```python
from build123d import *

# Parameters (mm, degrees)
EXTRUDE_1_DEPTH     = 10
CUT_EXTRUDE_1_REACH = 42.24
SKETCH_2_W          = 5
SKETCH_2_H          = 10


with BuildPart() as part:
    # 草圖1 → 伸長1 (new body)
    with BuildSketch(Plane.XY):
        with BuildLine():
            Line((-466, 20.12), (466, 20.12))
            ThreePointArc((466, 20.12), (486.12, 0), (466, -20.12))
            Line((466, -20.12), (-466, -20.12))
            ThreePointArc((-466, -20.12), (-486.12, 0), (-466, 20.12))
        make_face()
        with BuildLine():
            Line((-466, 18.62), (466, 18.62))
            ThreePointArc((466, 18.62), (484.62, 0), (466, -18.62))
            Line((466, -18.62), (-466, -18.62))
            ThreePointArc((-466, -18.62), (-484.62, 0), (-466, 18.62))
        make_face(mode=Mode.SUBTRACT)
    extrude(amount=EXTRUDE_1_DEPTH)

    # 草圖2 → 除料-伸長1 (cut, up to next)
    with BuildSketch(Plane(origin=(0, 20.12, 0), x_dir=(1, 0, 0), z_dir=(0, 1, 0)), mode=Mode.PRIVATE) as cut_extrude_1_sk1:
        with Locations((27.677656209, -5)):
            Rectangle(SKETCH_2_W, SKETCH_2_H)
    cut_extrude_1_tool1 = extrude(cut_extrude_1_sk1.sketch, amount=-CUT_EXTRUDE_1_REACH, mode=Mode.PRIVATE) & part.part
    add(cut_extrude_1_tool1.solids().sort_by_distance((27.677656, 20.12, 5))[0], mode=Mode.SUBTRACT)


solid = part.part
```
Verification items for the finished model (mm, model axes). A direction names the side the tool comes from. Coordinates: 2 decimals unless noted, no trailing zeros. Order: outer loops, then holes, each group sorted by start corner. A loop starts at its lowest first (then second) coordinate and runs counter-clockwise, first axis right, second up. Notation, with made-up numbers: (82, 26) - (86, 26) arc R19 ccw to (86, 54) - close; hole circle Ø2 at (85.5, 60.25). An arc over 180 degrees is marked (long way). Return JSON: item names as keys, results as strings.
(1) Section check C-C, the plane z = 5.75. Record the cut outline in (x, y), and give its area (3 significant figures).
Filled sheet:
{"outline": "(-466, -20.12) - (466, -20.12) arc R20.12 ccw to (466, 20.12) - (30.18, 20.12) - (30.18, 18.62) - (466, 18.62) arc R18.62 cw to (466, -18.62) - (-466, -18.62) arc R18.62 cw to (-466, 18.62) - (25.18, 18.62) - (25.18, 20.12) - (-466, 20.12) arc R20.12 ccw to start", "area": "2,970 mm^2"}
(2) Thickness scan on line 1 along X through (y, z) = (1.5, 4.75); line 2 along Y through (x, z) = (425.5, 5.5); line 3 along X through (y, z) = (-11, 1.5). Record the ranges inside material, lowest first.
Filled sheet:
{"line 1": "x = -486.06 to -484.56, 484.56 to 486.06", "line 2": "y = -20.12 to -18.62, 18.62 to 20.12", "line 3": "x = -482.85 to -481.02, 481.02 to 482.85"}
(3) Mould release check, pull along Y, two halves, no side actions. Record for faces 3 (the cylindrical face through (-484.615, -0.409, 4.93)), 4 (the cylindrical face through (-486.115, -0.442, 4.93)), 5 (the flat face through (2, 19, 10)): pulls with the +Y half, pulls with the -Y half, needs draft (parallel to the pull), parting line crosses it, or undercut.
Filled sheet:
{"face 3": "undercut", "face 4": "parting line crosses it", "face 5": "needs draft"}
(4) Go/stop test with flat-tipped pins: pin 1 (3 mm diameter, centred on y = -11, z = 3, fed in from +X); pin 2 (0.8 mm diameter, centred on y = 19, z = 3.5, fed in from -X); pin 3 (4 mm diameter, centred on y = -4, z = 2, fed in from +X). Record where each tip stops, or that it passes through.
Filled sheet:
{"pin 1": "stops at x = 483.74", "pin 2": "stops at x = -473.67", "pin 3": "stops at x = 486.02"}
(5) Section check B-B, the plane y = -3.5. Record the cut outline in (x, z), and give its area (3 significant figures).
Filled sheet:
{"outline": "(-485.81, 0) - (-484.29, 0) - (-484.29, 10) - (-485.81, 10) - close; (484.29, 0) - (485.81, 0) - (485.81, 10) - (484.29, 10) - close", "area": "30.5 mm^2"}
(6) Access from +Z, -Z, +X, -X, +Y, -Y to the whole of each face (thin tool, end or side, straight path). Record for faces 1 (the flat face through (2, 19, 0)), 2 (the cylindrical face through (484.615, 0.409, 4.93)).
Filled sheet:
{"face 1": "-Z, +X, -X, +Y, -Y", "face 2": "+Z, -Z"}
(7) Section check A-A, the plane x = 38. Record the cut outline in (y, z).
Filled sheet:
{"outline": "(-20.12, 0) - (-18.62, 0) - (-18.62, 10) - (-20.12, 10) - close; (18.62, 0) - (20.12, 0) - (20.12, 10) - (18.62, 10) - close"}
